Source: CAD feature listing. Evaluate the final solid. Frame: model axes, mm. A direction names the side the tool comes from. Give positions to 0.01 mm unless a question says otherwise; leave off trailing zeros. Order: outer loops, then holes, each group sorted by start corner. A loop starts at its lowest first (then second) coordinate and runs counter-clockwise, first axis right, second up. Notation, with made-up numbers: (-22.5, 57.5) - (24.5, 57.5) arc R8 cw to (24.5, 70.5) - close; hole circle Ø11 at (-5.75, -32). An arc over 180 degrees is marked (long way). Write each question's results on one line, items separated by ' | '. Start each with the question number.
Item 1: Section D-D on x = -21. Output: boundary loops of the cut face in (y, z), and give its area (3 significant figures).
Item 2: Section A-A on z = 23. Output: boundary loops of the cut face in (x, y).
Item 3: Section C-C on z = 60.5. Output: boundary loops of the cut face in (x, y).
Item 4: Section B-B on y = 128. Output: boundary loops of the cut face in (x, z).
Item 5: Line query: line 1 along X through (y, z) = (-56.5, 68); line 2 along Z through (x, y) = (0, -85.2); line 3 along Y through (x, z) = (-31.5, 8). Output: solid intervals per line, ascending.
Item 6: Contact query for flat-ended pins moving along their axis: pin 1 Ø22.5 at (x, y) = (-12, -58.5) entering from +Z; pin 2 Ø8 at (x, z) = (36, 8.5) entering from +Y; pin 3 Ø4 at (y, z) = (102, 5) entering from +X. Output: stop coordinate, or through.
Item 7: Mould query, pull axis Y, two halves, no side actions, for faces 1 (the flat face through (15.3, 123.2, 4.5)), 2 (the flat face through (-11, 128, 2)), 3 (the flat face through (-1, -87.5, 37)). Classes: released by +Y, released by -Y, zero draft, split by the parting line, or undercut.
Item 8: Set-up query: faces 4 (the flat face through (45, -1, 40)), 5 (the flat face through (-36, 97, 5)), 6 (the flat face through (36, 97, 5)), 7 (the flat face through (-15.7, 122.8, 4.5)). Return all of +Z, -Z, +X, -X, +Y, -Y with unobstructed straight access to the full face (end or side cutting, diameter ignored); none if empty.
```python
from build123d import *

# Parameters (mm, degrees)
SKETCH1_W           = 96
SKETCH1_H           = 175
BOSS_EXTRUDE1_DEPTH = 100
SKETCH2_W           = 90
SKETCH2_H           = 169
CUT_EXTRUDE1_DEPTH  = 87
SKETCH3_W           = 56.5
SKETCH3_H           = 164
CUT_EXTRUDE2_DEPTH  = 10
SKETCH5_R           = 6
CUT_EXTRUDE3_DEPTH  = 10
SKETCH6_W           = 33.5
SKETCH6_H           = 48
CUT_EXTRUDE4_DEPTH  = 10
CUT_EXTRUDE6_DEPTH  = 10
SKETCH10_W          = 96
SKETCH10_H          = 25
CUT_EXTRUDE8_DEPTH  = 200
FILLET1_R           = 2
SKETCH11_R          = 2.5
CUT_EXTRUDE9_DEPTH  = 5
SKETCH12_W          = 5
SKETCH12_H          = 5
BOSS_EXTRUDE2_DEPTH = 20
BOSS_EXTRUDE5_DEPTH = 5


with BuildPart() as part:
    # Sketch1 → Boss-Extrude1 (new body)
    with BuildSketch(Plane.XY):
        Rectangle(SKETCH1_W, SKETCH1_H)
    extrude(amount=BOSS_EXTRUDE1_DEPTH)

    # Sketch2 → Cut-Extrude1 (cut)
    with BuildSketch(Plane.XY.offset(100)):
        Rectangle(SKETCH2_W, SKETCH2_H)
    extrude(amount=-CUT_EXTRUDE1_DEPTH, mode=Mode.SUBTRACT)

    # Sketch3 → Cut-Extrude2 (cut)
    with BuildSketch(Plane.XY.offset(13)):
        with Locations((-16.75, 0)):
            Rectangle(SKETCH3_W, SKETCH3_H)
    extrude(amount=-CUT_EXTRUDE2_DEPTH, mode=Mode.SUBTRACT)

    # Sketch5 → Cut-Extrude3 (cut)
    with BuildSketch(Plane(origin=(0, -84.5, 0), x_dir=(1, 0, 0), z_dir=(0, 1, 0))):
        with Locations((28.25, -23)):
            Circle(SKETCH5_R)
    extrude(amount=-CUT_EXTRUDE3_DEPTH, mode=Mode.SUBTRACT)

    # Sketch6 → Cut-Extrude4 (cut)
    with BuildSketch(Plane.XY.offset(13)):
        with Locations((28.25, -15.5)):
            Rectangle(SKETCH6_W, SKETCH6_H)
    extrude(amount=-CUT_EXTRUDE4_DEPTH, mode=Mode.SUBTRACT)

    # Sketch9 → Cut-Extrude6 (cut)
    with BuildSketch(Plane.XZ.offset(-84.5)):
        with BuildLine():
            Line((13, 20), (28, 20))
            ThreePointArc((28, 20), (31.5, 16.5), (28, 13))
            Line((28, 13), (13, 13))
            ThreePointArc((13, 13), (9.5, 16.5), (13, 20))
        make_face()
    extrude(amount=-CUT_EXTRUDE6_DEPTH, mode=Mode.SUBTRACT)

    # Sketch10 → Cut-Extrude8 (cut)
    with BuildSketch(Plane.XZ.offset(87.5)):
        with Locations((0, 87.5)):
            Rectangle(SKETCH10_W, SKETCH10_H)
    extrude(amount=-CUT_EXTRUDE8_DEPTH, mode=Mode.SUBTRACT)

    # Fillet1
    fillet1_edges = [part.edges().sort_by_distance(p)[0] for p in [
        (0, 87.5, 0),
        (48, 0, 0),
        (0, -87.5, 0),
        (-48, 0, 0),
        (-48, 87.5, 37.5),
        (48, 87.5, 37.5),
        (48, -87.5, 37.5),
        (-48, -87.5, 37.5),
        (-48, 0, 75),
        (0, 87.5, 75),
        (48, 0, 75),
        (0, -87.5, 75),
    ]]
    fillet(fillet1_edges, radius=FILLET1_R)

    # Sketch11 → Cut-Extrude9 (cut)
    with BuildSketch(Plane.XZ.offset(87.5)):
        with Locations((0, 23)):
            Circle(SKETCH11_R)
    extrude(amount=-CUT_EXTRUDE9_DEPTH, mode=Mode.SUBTRACT)

    # Sketch12 → Boss-Extrude2 (add)
    with BuildSketch(Plane(origin=(0, 87.5, 0), x_dir=(1, 0, 0), z_dir=(0, 1, 0))):
        with Locations((-33.5, -4.5)):
            Rectangle(SKETCH12_W, SKETCH12_H)
        with Locations((33.5, -4.5)):
            Rectangle(SKETCH12_W, SKETCH12_H)
    extrude(amount=BOSS_EXTRUDE2_DEPTH)

    # Sketch15 → Boss-Extrude5 (add)
    with BuildSketch(Plane.XY.offset(7)):
        Polygon((-31, 107.5), (0, 138.5), (31, 107.5), (36, 107.5), (0, 143.5), (-36, 107.5), align=None)
    extrude(amount=-BOSS_EXTRUDE5_DEPTH)


solid = part.part
```
Evaluation:
1) outline: (-87.5, 2) arc R2 ccw to (-85.5, 0) - (85.5, 0) arc R2 ccw to (87.5, 2) - (87.5, 73) arc R2 ccw to (85.5, 75) - (84.5, 75) - (84.5, 13) - (82, 13) - (82, 3) - (-82, 3) - (-82, 13) - (-84.5, 13) - (-84.5, 75) - (-85.5, 75) arc R2 ccw to (-87.5, 73) - close; (117.5, 2) - (122.5, 2) - (122.5, 7) - (117.5, 7) - close | area: 1,030 mm^2
2) outline: (-48, -85.5) arc R2 ccw to (-46, -87.5) - (-2.5, -87.5) - (-2.5, -84.5) - (-45, -84.5) - (-45, 84.5) - (45, 84.5) - (45, -84.5) - (34.25, -84.5) - (34.25, -87.5) - (46, -87.5) arc R2 ccw to (48, -85.5) - (48, 85.5) arc R2 ccw to (46, 87.5) - (-46, 87.5) arc R2 ccw to (-48, 85.5) - close; (2.5, -87.5) - (22.25, -87.5) - (22.25, -84.5) - (2.5, -84.5) - close
3) outline: (-48, -85.5) arc R2 ccw to (-46, -87.5) - (46, -87.5) arc R2 ccw to (48, -85.5) - (48, 85.5) arc R2 ccw to (46, 87.5) - (-46, 87.5) arc R2 ccw to (-48, 85.5) - close; hole (-45, -84.5) - (45, -84.5) - (45, 84.5) - (-45, 84.5) - close
4) outline: (-15.5, 2) - (-10.5, 2) - (-10.5, 7) - (-15.5, 7) - close; (10.5, 2) - (15.5, 2) - (15.5, 7) - (10.5, 7) - close
5) line 1: x = -48 to -45, 45 to 48 | line 2: z = 0 to 20.5, 25.5 to 75 | line 3: y = -87.5 to -82, 82 to 87.5
6) pin 1: stops at z = 3 | pin 2: stops at y = 111.21 | pin 3: stops at x = 36
7) face 1: undercut | face 2: zero draft | face 3: released by -Y
8) face 4: +Z | face 5: +Z, -Z, -X, +Y | face 6: +Z, -Z, +X, +Y | face 7: +Z, -Z
